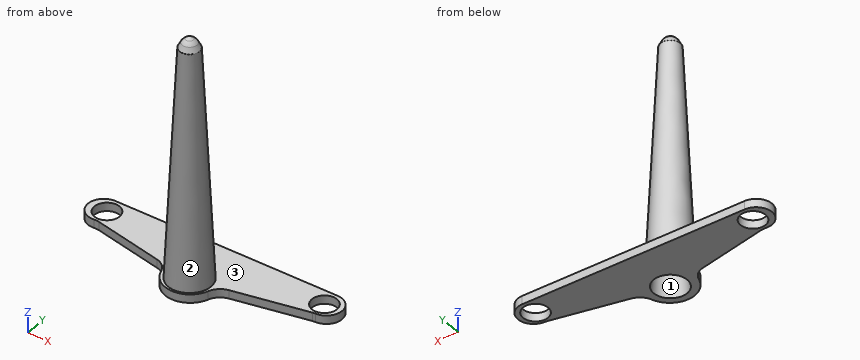
```python
from build123d import *

# Parameters (mm, degrees)
F0_R     = 2.25
F0_R_2   = 1.5
F1_DEPTH = 1
F2_R     = 2
F5_R     = 2
F6_DEPTH = 29.7303643356
F6_TAPER = 4
F7_R     = 1


with BuildPart() as f1:
    # F0 (on Top) → F1 (new body)
    with BuildSketch(Plane.XY):
        with BuildLine():
            Line((13.3969206363, 1.9189893501), (-13.6030793637, 1.9189893501))
            ThreePointArc((-13.6030793637, 1.9189893501), (-15.476354869, -0.2010418621), (-13.1418243737, -1.7990596423))
            Line((-13.1418243737, -1.7990596423), (-3.0734528816, -3.9087251454))
            ThreePointArc((-3.0734528816, -3.9087251454), (-0.0744018388, -7.0627152846), (2.9271771184, -3.9111308071))
            Line((2.9271771184, -3.9111308071), (13.3021756263, -1.7970976995))
            ThreePointArc((13.3021756263, -1.7970976995), (15.2555679655, 0.0123501208), (13.3969206363, 1.9189893501))
        make_face()
        with Locations((0, -4.3)):
            Circle(F0_R, mode=Mode.SUBTRACT)
        with Locations((-13.2, 0)):
            Circle(F0_R_2, mode=Mode.SUBTRACT)
        with Locations((13.2, 0)):
            Circle(F0_R_2, mode=Mode.SUBTRACT)
    extrude(amount=F1_DEPTH)

    # F2
    f2_edges = [f1.edges().sort_by_distance(p)[0] for p in [
        (2.927177, -3.911131, 0.5),
        (13.302176, -1.797098, 0.5),
        (-13.141824, -1.79906, 0.5),
        (-3.073453, -3.908725, 0.5),
    ]]
    fillet(f2_edges, radius=F2_R)

    # F3 (on Right) → F4 (revolve)
    with BuildSketch(Plane.YZ):
        Polygon((-4.2690001428, 0), (-1.6726437025, 0), (-3.0743933748, 28.4580495209), (-3.5435410682, 29.3574947864), (-4.2690001428, 29.7293643356), align=None)
    revolve(axis=Axis((0, -4.2690001428, 17.7293643356), (0, 0, 1)))

    # F5 (on face) → F6 (cut, through all)
    with BuildSketch(Plane.XY):
        with Locations((0, -4.2691347189)):
            Circle(F5_R)
    extrude(amount=F6_DEPTH, taper=F6_TAPER, mode=Mode.SUBTRACT)

    # F7
    f7_edges = [f1.edges().sort_by_distance(p)[0] for p in [
        (0, -4.994459, 29.357495),
    ]]
    fillet(f7_edges, radius=F7_R)


solid = f1.part
```
Here's how the part is built. I have some questions about the finished solid (model axes, mm). Face numbers are marked on the shaded views. Give positions to 0.01 mm unless a question says otherwise; leave off trailing zeros. Write each loop counter-clockwise with the first axis right and the second up, starting at its lowest first coordinate (ties: lowest second). Pieces come first, ordered by that corner, then holes. Notation, with made-up numbers: M 61.5,47 L 88.5,47 A25 cw 88.5,82 Z; hole C 58,11.5 d7. An arc over 180 degrees is marked long. Put each result on its own line as item: value. Start each with the question number.
Item 1: If we section it at A-A, the plane y = 0: Write out the boundary of the cut face in (x, z).
Item 2: Will these pins go through, and if not, where does the flat tip stop? pin 1 (1.5 mm diameter, centred on x = -2, z = 12, fed in from -Y); pin 2 (1.5 mm diameter, centred on y = -1.5, z = 4, fed in from +X); pin 3 (3.5 mm diameter, centred on x = -13.2, y = 0, fed in from -Z).
Item 3: If we section it at C-C, the plane x = 8.5: Write out the boundary of the cut face in (y, z).
Item 4: If we section it at B-B, the plane z = 21.5: Write out the boundary of the cut face in (x, y), then the cut area to 3 significant figures.
Item 5: Thinking about a two-plate mould opening in Y: for the marked faces 1, 2 and 3, which applies, +Y half, -Y half, draft (parallel to the pull), parting line (faces both ways), or undercut?
Item 6: I need wall thicknesses on L1, parallel to Y at x = -13.2, z = 0.65; L2, parallel to Z at x = 10.5, y = -1; L3, parallel to X at y = -4.5, z = 9.75. Which ranges of each line are inside material? Lowest first, please. Write a range as from..to.
Item 7: If we section it at D-D, the plane z = 16.25: Write out the boundary of the cut face in (x, y).
Values:
1. outline: M -15.49,0 L -14.7,0 L -14.7,1 L -15.49,1 Z; M -11.7,0 L 11.7,0 L 11.7,1 L -11.7,1 Z; M 14.7,0 L 15.26,0 L 15.26,1 L 14.7,1 Z
2. pin 1: y = -5.84
2. pin 2: x = 1.3
2. pin 3: z = 0
3. outline: M -2.78,0 L 1.92,0 L 1.92,1 L -2.78,1 Z
4. outline: C 0,-4.27 d3.07; hole C 0,-4.27 d0.99
4. area: 6.65 mm²
5. face 1: undercut
5. face 2: parting line
5. face 3: draft
6. L1: -1.83..-1.5, 1.5..1.92
6. L2: 0..1
6. L3: -2.1..-1.3, 1.3..2.1
7. outline: C 0,-4.27 d3.59; hole C 0,-4.27 d1.73
